from build123d import *

# Parameters (mm, degrees)
BOSS_EXTRUDE1_DEPTH = 1.524
SKETCH1_3_R         = 1.2
BOSS_EXTRUDE2_DEPTH = 4.064
SKETCH1_4_R         = 1
SKETCH1_4_R_2       = 1.2
BOSS_EXTRUDE3_DEPTH = 6.35
SKETCH3_W           = 9.525
SKETCH3_H           = 3.175
BOSS_EXTRUDE4_DEPTH = 1.524
CHAMFER1_SIZE       = 1.524
BOSS_EXTRUDE5_START = -57
BOSS_EXTRUDE5_DEPTH = 57
CUT_EXTRUDE1_DEPTH  = 35.815330499
SKETCH6_W           = 17.468754951
SKETCH6_H           = 9.652
CUT_EXTRUDE2_DEPTH  = 35.815330499
BOSS_EXTRUDE6_DEPTH = 10.16


with BuildPart() as part:
    # Sketch1 → Boss-Extrude1 (new body)
    with BuildSketch(Plane(origin=(0, 0, 0), x_dir=(-1, 0, 0), z_dir=(0, 0, 1))):
        Polygon((11.893796958, -28.509907181), (11.893796958, 28.490092819), (-11.893796958, 28.490092819), (-11.893796958, -28.509907181), (-6.893796958, -23.509907181), (6.893796958, -23.509907181), align=None)
    extrude(amount=BOSS_EXTRUDE1_DEPTH)

    # Sketch1<3> → Boss-Extrude2 (add)
    # profile 1 of 4: a face of its own
    with BuildSketch(Plane(origin=(0, 0, 0), x_dir=(-1, 0, 0), z_dir=(0, 0, 1))):
        with BuildLine():
            ThreePointArc((-8.89, -17.709907181), (-11.69, -20.509907181), (-8.89, -23.309907181))
            Line((-8.89, -23.309907181), (-5.85, -23.309907181))
            Line((-5.85, -23.309907181), (-5.85, -17.709907181))
            Line((-5.85, -17.709907181), (-8.89, -17.709907181))
        make_face()
        with Locations(Location((-8.89, -20.509907181, 0), (0, 0, 180))):
            Circle(SKETCH1_3_R, mode=Mode.SUBTRACT)
    # profile 2 of 4: a face of its own
    with BuildSketch(Plane(origin=(0, 0, 0), x_dir=(-1, 0, 0), z_dir=(0, 0, 1))):
        with BuildLine():
            ThreePointArc((8.89, -23.309907181), (11.69, -20.509907181), (8.89, -17.709907181))
            Line((8.89, -17.709907181), (5.85, -17.709907181))
            Line((5.85, -17.709907181), (5.85, -23.309907181))
            Line((5.85, -23.309907181), (8.89, -23.309907181))
        make_face()
    # profile 3 of 4: a face of its own
    with BuildSketch(Plane(origin=(0, 0, 0), x_dir=(-1, 0, 0), z_dir=(0, 0, 1))):
        with BuildLine():
            ThreePointArc((7.89, 23.138861301), (11.19, 25.210092819), (7.89, 27.281324337))
            Line((7.89, 27.281324337), (7.89, 23.138861301))
        make_face()
    # profile 4 of 4: a face of its own
    with BuildSketch(Plane(origin=(0, 0, 0), x_dir=(-1, 0, 0), z_dir=(0, 0, 1))):
        with BuildLine():
            ThreePointArc((-7.89, 27.281324337), (-11.19, 25.210092819), (-7.89, 23.138861301))
            Line((-7.89, 23.138861301), (-7.89, 27.281324337))
        make_face()
    extrude(amount=-BOSS_EXTRUDE2_DEPTH)

    # Sketch1<4> → Boss-Extrude3 (add)
    with BuildSketch(Plane(origin=(0, 0, 0), x_dir=(-1, 0, 0), z_dir=(0, 0, 1))):
        with Locations(Location((8.89, 25.210092819, 0), (0, 0, 180))):
            Circle(SKETCH1_4_R)
        with Locations(Location((-8.89, -20.509907181, 0), (0, 0, 180))):
            Circle(SKETCH1_4_R_2)
        with Locations(Location((-8.89, 25.210092819, 0), (0, 0, 180))):
            Circle(SKETCH1_4_R)
        with Locations(Location((8.89, -20.509907181, 0), (0, 0, 180))):
            Circle(SKETCH1_4_R_2)
    extrude(amount=-BOSS_EXTRUDE3_DEPTH)

    # Sketch3 → Boss-Extrude4 (add)
    with BuildSketch(Plane(origin=(0, 0, 0), x_dir=(-1, 0, 0), z_dir=(0, 0, -1))):
        with Locations((0, 16.122407181)):
            Rectangle(SKETCH3_W, SKETCH3_H)
    extrude(amount=BOSS_EXTRUDE4_DEPTH)

    # Chamfer1
    chamfer1_edges = [part.edges().sort_by_distance(p)[0] for p in [
        (0, 14.534907181, -1.524),
    ]]
    chamfer(chamfer1_edges, length=CHAMFER1_SIZE - 0.0001)  # a hair under: the kernel refuses the full size

    # Sketch4 → Boss-Extrude5 (add)
    with BuildSketch(Plane.XZ.offset(28.490092819).offset(BOSS_EXTRUDE5_START)):
        with BuildLine():
            ThreePointArc((13.155591368, -1.15943863), (13.351412917, -6.186799511), (11.692856631, -10.936735779))
            Line((11.692856631, -10.936735779), (13.772671764, -12.084238841))
            ThreePointArc((13.772671764, -12.084238841), (15.831522609, -5.363460963), (14.786599753, 1.5875))
            Line((14.786599753, 1.5875), (-14.786599753, 1.5875))
            ThreePointArc((-14.786599753, 1.5875), (-15.829296194, -5.393105445), (-13.743006885, -12.135765541))
            Line((-13.743006885, -12.135765541), (-11.685926468, -10.948731172))
            ThreePointArc((-11.685926468, -10.948731172), (-13.350386295, -6.193649708), (-13.155591368, -1.15943863))
            Line((-13.155591368, -1.15943863), (-11.893796958, 0))
            Line((-11.893796958, 0), (11.893796958, 0))
            Line((11.893796958, 0), (13.155591368, -1.15943863))
        make_face()
    extrude(amount=BOSS_EXTRUDE5_DEPTH)

    # Sketch5 → Cut-Extrude1 (cut, through all)
    with BuildSketch(Plane(origin=(0, 0, 0), x_dir=(-1, 0, 0), z_dir=(0, 0, -1))):
        Polygon((11.893796958, 28.509907181), (-11.893796958, 28.509907181), (-6.893796958, 23.509907181), (6.893796958, 23.509907181), align=None)
    extrude(amount=-CUT_EXTRUDE1_DEPTH, mode=Mode.SUBTRACT)

    # Sketch6 → Cut-Extrude2 (cut, through all)
    with BuildSketch(Plane(origin=(0, 0, 0), x_dir=(0, 0, -1), z_dir=(1, 0, 0))):
        with Locations((11.782377476, 10.983907181)):
            Rectangle(SKETCH6_W, SKETCH6_H)
    extrude(amount=-CUT_EXTRUDE2_DEPTH, mode=Mode.SUBTRACT)

    # Sketch7 → Boss-Extrude6 (add)
    with BuildSketch(Plane(origin=(0, 0, 0), x_dir=(1, 0, 0), z_dir=(0, 1, 0))):
        with BuildLine():
            Line((-13.334610111, 6.296055118), (-11.933690156, 7.696975073))
            Line((-11.933690156, 7.696975073), (-10.802177885, 6.565462802))
            Line((-10.802177885, 6.565462802), (-13.496254721, 3.871385965))
            ThreePointArc((-13.496254721, 3.871385965), (-13.394733651, 2.5067686), (-13.155591368, 1.15943863))
            Line((-13.155591368, 1.15943863), (-11.893796958, 0))
            Line((-11.893796958, 0), (11.893796958, 0))
            Line((11.893796958, 0), (13.155591368, 1.15943863))
            ThreePointArc((13.155591368, 1.15943863), (13.394733651, 2.5067686), (13.496254721, 3.871385965))
            Line((13.496254721, 3.871385965), (10.802177885, 6.565462802))
            Line((10.802177885, 6.565462802), (11.933690156, 7.696975073))
            Line((11.933690156, 7.696975073), (13.334610111, 6.296055118))
            ThreePointArc((13.334610111, 6.296055118), (12.727038231, 8.691857223), (11.692856631, 10.936735779))
            Line((11.692856631, 10.936735779), (13.772671764, 12.084238841))
            ThreePointArc((13.772671764, 12.084238841), (15.831522609, 5.363460963), (14.786599753, -1.5875))
            Line((14.786599753, -1.5875), (-14.786599753, -1.5875))
            ThreePointArc((-14.786599753, -1.5875), (-15.829296194, 5.393105445), (-13.743006885, 12.135765541))
            Line((-13.743006885, 12.135765541), (-11.685926468, 10.948731172))
            ThreePointArc((-11.685926468, 10.948731172), (-12.724726374, 8.698386731), (-13.334610111, 6.296055118))
        make_face()
    extrude(amount=-BOSS_EXTRUDE6_DEPTH)


solid = part.part
Verification items for the finished model (mm, model axes). A direction names the side the tool comes from. Round coordinates to 2 decimals unless told otherwise and drop trailing zeros. Loops run counter-clockwise (first coordinate to the right, second up) from the corner with the lowest first, then second, coordinate; pieces in that order, holes last. Notation, with made-up numbers: (-10.75, -26) - (20.25, -26) arc R17 cw to (20.25, -3) - close; hole circle Ø2 at (25.25, 50.5). An arc over 180 degrees is marked (long way). Answer in a Markdown table with one row per item. Add a question column.
Q1. Gauge pin test, flat ends, axial feed: pin 1 (12 mm diameter, centred on x = 4, y = -8.5, fed in from -Z); pin 2 (2 mm diameter, centred on y = 19, z = -1.5, fed in from -X); pin 3 (1.6 mm diameter, centred on x = 10.5, y = -24, fed in from -Z). Record the tip position at first contact, or that the pin passes through.
Q2. Section check B-B on z = -10.25. Enter the section's corners in (x, y).
Q3. Material ranges on line 1 (X direction, y = -21, z = -4.25); line 2 (Z direction, x = 14, y = 20); line 3 (Z direction, x = 6, y = 1.5), recorded low to high.
Q4. Tool access check on faces 1 (the face through (-9, -25, -6.35)), 2 (the face through (-9.15, 19.34, -5.19)), 3 (the face through (11.36, -5.009, -7.123)). Record the directions out of +Z, -Z, +X, -X, +Y, -Y that give a thin tool (end or side, any length) a straight path to the whole face; none if there is none.
Q5. Release check for a two-part mould opening along X. For faces 4 (the face through (-15, 11, -3.048)), 5 (the face through (9, -25, -6.35)), 6 (the face through (-15.837, 0.409, -5.294)) record: pulls with the +X half, pulls with the -X half, needs draft (parallel to the pull), parting line crosses it, or undercut.
Found:
| question | item | result |
|---|---|---|
| 1 | pin 1 | stops at z = 0 |
| 1 | pin 2 | stops at x = -15.78 |
| 1 | pin 3 | stops at z = -4.06 |
| 2 | outline | (-14.67, -28.49) - (-12.06, -28.49) - (-12.06, 6.16) - (-14.67, 6.16) - close; (-14.67, 15.81) - (-12.06, 15.81) - (-12.06, 28.51) - (-14.67, 28.51) - close; (12.06, -28.49) - (14.67, -28.49) - (14.67, 28.51) - (12.06, 28.51) - close |
| 3 | line 1 | x = -15.87 to -13.5, 13.5 to 15.87 |
| 3 | line 2 | z = -11.67 to 1.59 |
| 3 | line 3 | z = 0 to 1.59 |
| 4 | face 1 | -Z, +Y, -Y |
| 4 | face 2 | -Z |
| 4 | face 3 | +Y, -Y |
| 5 | face 4 | needs draft |
| 5 | face 5 | undercut |
| 5 | face 6 | pulls with the -X half |
